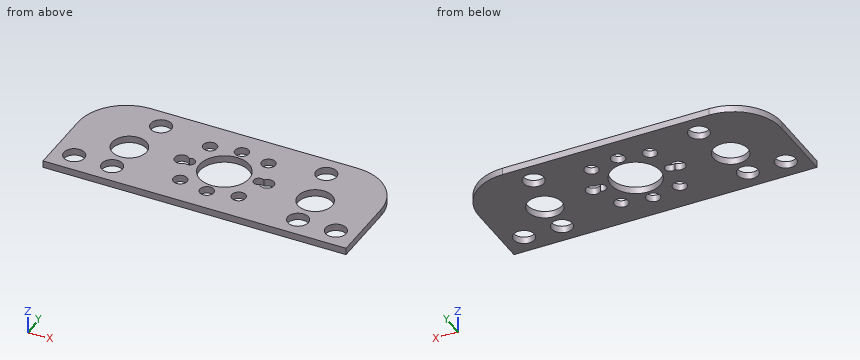
from build123d import *

# Parameters (mm, degrees)
EXTRUDE_1_DEPTH     = 1
SKETCH_6_R          = 1
SKETCH_6_R_2        = 3.6
CUT_EXTRUDE_1_DEPTH = 2
SKETCH_8_R          = 2.5
CUT_EXTRUDE_2_DEPTH = 2
SKETCH_12_R         = 1.5
CUT_EXTRUDE_3_DEPTH = 10


with BuildPart() as part:
    # 草图10 → 凸台-拉伸1 (new body)
    with BuildSketch(Plane.XY):
        with BuildLine():
            Line((-15, 8.5), (15, 8.5))
            ThreePointArc((15, 8.5), (19.949747468, 6.449747468), (22, 1.5))
            Line((22, 1.5), (22, -8.5))
            Line((22, -8.5), (-22, -8.5))
            Line((-22, -8.5), (-22, 1.5))
            ThreePointArc((-22, 1.5), (-19.949747468, 6.449747468), (-15, 8.5))
        make_face()
    extrude(amount=-EXTRUDE_1_DEPTH)

    # 草图6 → 切除-拉伸1 (cut)
    with BuildSketch(Plane.XY):
        with Locations((0, 5)):
            Circle(SKETCH_6_R)
        with Locations((0, -5)):
            Circle(SKETCH_6_R)
        Circle(SKETCH_6_R_2)
        with Locations((-4.242640687, 4.242640687)):
            Circle(SKETCH_6_R)
        with Locations((4.242640687, 4.242640687)):
            Circle(SKETCH_6_R)
        with Locations((-4.242640687, -4.242640687)):
            Circle(SKETCH_6_R)
        with Locations((4.242640687, -4.242640687)):
            Circle(SKETCH_6_R)
        with BuildLine():
            ThreePointArc((-5.417708333, -0.622912312), (-4.25, 0), (-5.417708333, 0.622912312))
            ThreePointArc((-5.417708333, 0.622912312), (-7.2, 0), (-5.417708333, -0.622912312))
        make_face()
        with BuildLine():
            ThreePointArc((5.417708333, 0.622912312), (4.25, 0), (5.417708333, -0.622912312))
            ThreePointArc((5.417708333, -0.622912312), (7.2, 0), (5.417708333, 0.622912312))
        make_face()
    extrude(amount=-CUT_EXTRUDE_1_DEPTH, mode=Mode.SUBTRACT)

    # 草图8 → 切除-拉伸2 (cut)
    with BuildSketch(Plane.XY):
        with Locations((-13.486660076, -0.6)):
            Circle(SKETCH_8_R)
        with Locations((13.486660076, -0.6)):
            Circle(SKETCH_8_R)
    extrude(amount=-CUT_EXTRUDE_2_DEPTH, mode=Mode.SUBTRACT)

    # 草图12 → 切除-拉伸3 (cut)
    with BuildSketch(Plane.XY):
        with Locations((-19, -5.5)):
            Circle(SKETCH_12_R)
        with Locations((19, -5.5)):
            Circle(SKETCH_12_R)
        with Locations((-12, 5.5)):
            Circle(SKETCH_12_R)
        with Locations((12, 5.5)):
            Circle(SKETCH_12_R)
        with Locations((-13.490737563, -5.5)):
            Circle(SKETCH_12_R)
        with Locations((13.5, -5.5)):
            Circle(SKETCH_12_R)
    extrude(amount=-CUT_EXTRUDE_3_DEPTH, mode=Mode.SUBTRACT)


solid = part.part
Model file for the job. Use its own axes, mm. Give positions to 0.01 mm unless a question says otherwise; leave off trailing zeros. Write each loop counter-clockwise with the first axis right and the second up, starting at its lowest first coordinate (ties: lowest second). Pieces come first, ordered by that corner, then holes. Notation, with made-up numbers: M 57.5,87 L 105.5,87 A13 ccw 105.5,112 Z; hole C -37.75,74.25 d1. An arc over 180 degrees is marked long. One line per item, written item: value. Start each with the question number.
Q1. Saw through at A-A, the plane x = 0. Write the cut outline in (y, z).
Q2. Drop flat-ended pins along their axis: pin 1 Ø1.6 at (x, y) = (6.2, 0) entering from -Z; pin 2 Ø6 at (x, y) = (-15.5, 5.5) entering from +Z. Give the stop position or say it passes through.
Q3. Saw through at B-B, the plane x = 18. Write the cut outline in (y, z), plus the area to 3 significant figures.
Q4. Saw through at C-C, the plane z = -0.8. State how many separate pieces and enclosed holes the cut face has, plus the area to 3 significant figures.
Q5. Probe probe 1 along Y at (x, z) = (0, -0.45); probe 2 along Y at (x, z) = (-4.5, -0.85); probe 3 along X at (y, z) = (-2, -0.15). List the from-to ranges inside material, lowest first. Write a range as [from, to].
Output values:
1. outline: M -8.5,-1 L -6,-1 L -6,0 L -8.5,0 Z; M -4,-1 L -3.6,-1 L -3.6,0 L -4,0 Z; M 3.6,-1 L 4,-1 L 4,0 L 3.6,0 Z; M 6,-1 L 8.5,-1 L 8.5,0 L 6,0 Z
2. pin 1: passes through
2. pin 2: stops at z = 0
3. outline: M -8.5,-1 L -6.62,-1 L -6.62,0 L -8.5,0 Z; M -4.38,-1 L 7.82,-1 L 7.82,0 L -4.38,0 Z
3. area: 14.1 mm²
4. separate pieces: 1
4. enclosed holes: 17
4. area: 577 mm²
5. probe 1: y = [-8.5, -6], [-4, -3.6], [3.6, 4], [6, 8.5]
5. probe 2: y = [-8.5, -5.21], [-3.28, -0.56], [0.56, 3.28], [5.21, 8.5]
5. probe 3: x = [-22, -15.56], [-11.42, -2.99], [2.99, 11.42], [15.56, 22]
